The model under review builds one solid part; all positions refer to its coordinate system, in mm. Face numbers are marked on the shaded views. A direction names the side the tool comes from. Coordinates: 2 decimals unless noted, no trailing zeros. Write each loop counter-clockwise with the first axis right and the second up, starting at its lowest first coordinate (ties: lowest second). Pieces come first, ordered by that corner, then holes. Notation, with made-up numbers: (13.25, 7.25) - (42.25, 7.25) arc R28 ccw to (42.25, 38.25) - close; hole circle Ø4 at (73.5, -2.5). An arc over 180 degrees is marked (long way). Put each result on its own line as item: value.
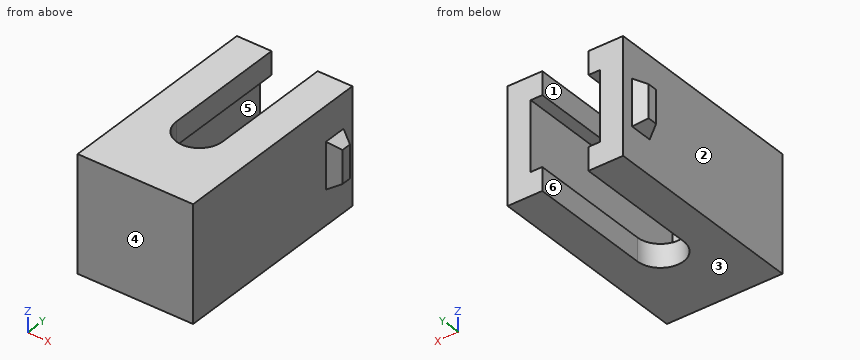
Autodesk Inventor part; units mm, degrees
ref_plane "YZ Plane" through (0, 0, 0) normal (1, 0, 0) x (0, 1, 0)
ref_plane "XZ Plane" through (0, 0, 0) normal (0, 1, 0) x (-1, 0, 0)
ref_plane "XY Plane" through (0, 0, 0) normal (0, 0, 1) x (1, 0, 0)
sketch "Sketch1" plane through (0, 0, 0) normal (0, 1, 0) x (-1, 0, 0)
  line L0 (-2.5, 2.5) -> (2.5, 2.5)
  line L1 (2.5, 2.5) -> (2.5, -2.5)
  line L2 (2.5, -2.5) -> (-2.5, -2.5)
  line L3 (-2.5, -2.5) -> (-2.5, 2.5)
  line L4 (-2.5, 2.5) -> (2.5, -2.5) construction
  line L5 (2.5, 2.5) -> (-2.5, -2.5) construction
  point P0 (0, 0)
  dimension "d0" = 5
  dimension "d1" = 5
extrude "Extrusion1" add sketch "Sketch1" along normal blind 9
shell "Shell1" thickness 1 removed faces 1 at (-0.8333, 9, -0.8333)
sketch "Sketch9" plane through (2.5, 0, 2.5) normal (1, 0, 0) x (0, 0, -1)
  line L0 (1.5, 7.5) -> (3.5, 7.5)
  line L1 (3.5, 7.5) -> (3.5, 8.5)
  line L2 (3.5, 8.5) -> (1.5, 8.5)
  line L3 (1.5, 8.5) -> (1.5, 7.5)
  line L4 (1.5, 7.5) -> (3.5, 8.5) construction
  line L5 (3.5, 7.5) -> (1.5, 8.5) construction
  line L6 (0, 9) -> (5, 9)
  point P0 (2.5, 0)
  point P1 (2.5, 8)
  dimension "d10" = 1
  dimension "d14" = 2
  dimension "d15" = 1
extrude "Extrusion4" add sketch "Sketch9" along normal blind 0.5 draft -30
sketch "Sketch10" plane through (-2.5, 0, -2.5) normal (-1, 0, 0) x (0, 0, 1)
  line L0 (1.5, 7.5) -> (3.5, 7.5)
  line L1 (3.5, 7.5) -> (3.5, 8.5)
  line L2 (3.5, 8.5) -> (1.5, 8.5)
  line L3 (1.5, 8.5) -> (1.5, 7.5)
  line L4 (1.5, 7.5) -> (3.5, 8.5) construction
  line L5 (3.5, 7.5) -> (1.5, 8.5) construction
  line L6 (0, 9) -> (5, 9)
  point P0 (2.5, 0)
  point P1 (2.5, 8)
  dimension "d13" = 1
  dimension "d16" = 2
  dimension "d17" = 1
extrude "Extrusion5" add sketch "Sketch10" along normal blind 0.5 draft -30
sketch "Sketch11" plane through (2.5, 0, -2.5) normal (0, 0, -1) x (-1, 0, 0)
  line L0 (2.5, 7.862) -> (2.5, 3.6245) construction
  line L1 (1.5, 7.862) -> (1.5, 3.6245)
  line L2 (3.5, 3.6245) -> (3.5, 7.862)
  arc A0 (3.5, 7.862) -> (1.5, 7.862) centre (2.5, 7.862) ccw
  arc A1 (1.5, 3.6245) -> (3.5, 3.6245) centre (2.5, 3.6245) ccw
  point P0 (2.5, 0)
  point P1 (2.5, 5.7432)
  dimension "d20" = 2
extrude "Extrusion6" cut sketch "Sketch11" against normal through all
sketch "Sketch12" plane through (2.5, 0, -2.5) normal (0, 0, -1) x (-1, 0, 0)
  line L0 (1.5, 7.862) -> (1.5, 3.6245)
  line L1 (1.5, 7.862) -> (3.5, 7.862)
  line L2 (3.5, 7.862) -> (3.5, 10.4679)
  line L3 (3.5, 10.4679) -> (1.5, 10.4679)
  line L4 (1.5, 10.4679) -> (1.5, 7.862)
  point P0 (2.5, 0)
  dimension "d23" = 2
extrude "Extrusion7" cut sketch "Sketch12" against normal through all
equation "\"d16\" = d14"
equation "\"d17\" = d15"
properties part number "snapfit_part_v04"
1. Machinability: for the marked faces 4, 5 and 6, which of the approach directions +Z, -Z, +X, -X, +Y, -Y give a long, thin tool a straight path to every point of the face, cutting with its end or side? Answer none if there is none.
Determined:
face 4: +Z, -Z, +X, -X, -Y
face 5: +Y
face 6: +Z, -Z, +Y
2. Consider section C-C on x = 0. State the section outline as (y, z) points, plus the area to 3 significant figures.
Determined:
outline: (0, -2.5) - (2.62, -2.5) - (2.62, -1.5) - (1, -1.5) - (1, 1.5) - (2.62, 1.5) - (2.62, 2.5) - (0, 2.5) - close
area: 8.25 mm^2
3. Consider section B-B on z = 1.3. State the section outline as (x, y) points.
Determined:
outline: (-2.5, 0) - (2.5, 0) - (2.5, 9) - (1.5, 9) - (1.5, 1) - (-1.5, 1) - (-1.5, 9) - (-2.5, 9) - close
4. The part is to be moulded in two halves that separate along X. For the marked faces 1, 2 and 3, say which applies: +X half, -X half, draft (parallel to the pull), parting line (faces both ways), or undercut.
Determined:
face 1: undercut
face 2: -X half
face 3: draft
5. Consider section A-A on y = 6.5. State the section outline as (x, z) points.
Determined:
outline: (-2.5, -2.5) - (-1, -2.5) - (-1, -1.5) - (-1.5, -1.5) - (-1.5, 1.5) - (-1, 1.5) - (-1, 2.5) - (-2.5, 2.5) - close; (1, -2.5) - (2.5, -2.5) - (2.5, 2.5) - (1, 2.5) - (1, 1.5) - (1.5, 1.5) - (1.5, -1.5) - (1, -1.5) - close
6. For pin 1 Ø1.5 at (y, z) = (4, 0) entering from -X; pin 2 Ø2.5 at (y, z) = (4.5, 0) entering from +X; pin 3 Ø3.5 at (x, y) = (0.5, 4.5) entering from +Z, all flat-tipped, find the tip position at first contact; note any pin that passes through.
Determined:
pin 1: stops at x = -2.5
pin 2: stops at x = 2.5
pin 3: stops at z = 2.5
7. Consider section D-D on y = 2.75. State the section outline as (x, z) points, plus the area to 3 significant figures.
Determined:
outline: (-2.5, -2.5) - (-0.49, -2.5) - (-0.49, -1.5) - (-1.5, -1.5) - (-1.5, 1.5) - (-0.49, 1.5) - (-0.49, 2.5) - (-2.5, 2.5) - close; (0.49, -2.5) - (2.5, -2.5) - (2.5, 2.5) - (0.49, 2.5) - (0.49, 1.5) - (1.5, 1.5) - (1.5, -1.5) - (0.49, -1.5) - close
area: 14.1 mm^2
8. To check wall thickness, follow probe 1 along X at (y, z) = (8.5, -1.1); probe 2 along X at (y, z) = (6.25, -2). State the ranges of each line that lie inside material, in increasing order.
Determined:
probe 1: x = -2.5 to -1.5, 1.5 to 2.5
probe 2: x = -2.5 to -1, 1 to 2.5
